Here's how the part is built. I have some questions about the finished solid (model axes, mm). A direction names the side the tool comes from. Coordinates: 2 decimals unless noted, no trailing zeros. Loops run counter-clockwise (first coordinate to the right, second up) from the corner with the lowest first, then second, coordinate; pieces in that order, holes last. Notation, with made-up numbers: (-23, -18) -> (-18, -18) arc R26 cw to (-18, 15) -> close; hole circle Ø7 at (21, -11.75). An arc over 180 degrees is marked (long way). Answer as a JSON object with one key per item and string values. Group by question number.
Q1. I want a section at A-A on z = 5. Count the separate pieces of the cut face and the enclosed holes in it, then the cut area to 3 significant figures.
Q2. I need wall thicknesses on line 1 (Z direction, x = -20.55, y = 65); line 2 (Y direction, x = -17.75, z = 3.5); line 3 (X direction, y = 22, z = 3.75). Which ranges of each line are inside material? Lowest first, please.
Q3. Thinking about a two-plate mould opening in Z: for faces 4 (the flat face through (-14, 39, 10)), 5 (the cylindrical face through (-19.96, 71.9, 5.09)), 6 (the flat face through (-17, 67, 3)), which applies, released by +Z, released by -Z, zero draft, split by the parting line, or undercut?
Q4. I'm going to push flat-ended pins straight in: pin 1 (3 mm diameter, centred on y = 40, z = 5.5, fed in from -X); pin 2 (3.5 mm diameter, centred on y = 65, z = 5, fed in from +X); pin 3 (6 mm diameter, centred on y = 21.5, z = 6, fed in from -X). Where does each tip first touch, or does it pass through?
Q5. On a 3-axis mill with a long thin cutter (end or side, diameter ignored), from which of +Z, -Z, +X, -X, +Y, -Y can I reach the whole of each face in a straight line? I mean faces 1 (the flat face through (-15, 20, 5)), 2 (the flat face through (-9.789, 2.098, 4.93)), 3 (the cylindrical face through (-22.4, 79.43, 5.07)). Say none if no direction works.
Q6. I want a section at C-C on x = -17.75. Write out the boundary of the cut face in (y, z).
Q7. I want a section at B-B on y = 66. Write out the boundary of the cut face in (x, z).
```python
from build123d import *

# Parameters (mm, degrees)
EXTRUDE_1_DEPTH     = 10
SKETCH_2_R          = 2.1
CUT_EXTRUDE_1_DEPTH = 82.018516402
SKETCH_3_R          = 0.8
CUT_EXTRUDE_2_DEPTH = 84.839131675
FILLET_1_R          = 0.5
FILLET_2_R          = 2


with BuildPart() as part:
    # 草图1 → 凸台-拉伸1 (new body)
    with BuildSketch(Plane.XY):
        Polygon((-9, 3.464101615), (-11, 0), (-9, -3.464101615), (-15, -3.464101615), (-15, 41.143593539), (-23, 55), (-23, 80), (-17, 80), (-17, 54.607695155), (-9, 40.751288694), align=None)
    extrude(amount=EXTRUDE_1_DEPTH)

    # 草图2 → 切除-拉伸1 (cut, through all)
    with BuildSketch(Plane(origin=(-17, 0, 0), x_dir=(0, 0, -1), z_dir=(1, 0, 0))):
        with Locations(Location((-5, 65, 0), (0, 0, 90))):
            Circle(SKETCH_2_R)
        with Locations(Location((-5, 74, 0), (0, 0, 90))):
            Circle(SKETCH_2_R)
    extrude(amount=-CUT_EXTRUDE_1_DEPTH, mode=Mode.SUBTRACT)

    # 草图3 → 切除-拉伸2 (cut, through all)
    with BuildSketch(Plane.XY.offset(10)):
        with Locations((-10.2, 0)):
            Circle(SKETCH_3_R)
        Polygon((-15, -1.07179677), (-13.618802154, -3.464101615), (-15, -3.464101615), align=None)
    extrude(amount=-CUT_EXTRUDE_2_DEPTH, mode=Mode.SUBTRACT)

    # 圆角1
    fillet_1_edges = [part.edges().sort_by_distance(p)[0] for p in [
        (-9, -3.464101615, 5),
        (-15, -1.07179677, 5),
        (-13.618802154, -3.464101615, 5),
    ]]
    fillet(fillet_1_edges, radius=FILLET_1_R)

    # 圆角2
    fillet_2_edges = [part.edges().sort_by_distance(p)[0] for p in [
        (-15, 41.143593539, 5),
        (-23, 55, 5),
        (-23, 80, 5),
        (-17, 80, 5),
        (-17, 54.607695155, 5),
        (-9, 40.751288694, 5),
    ]]
    fillet(fillet_2_edges, radius=FILLET_2_R)


solid = part.part
```
Result set:
{
 "1": {"separate pieces": "3", "enclosed holes": "0", "area": "437 mm²"},
 "2": {"line 1": "z = 0 to 2.9, 7.1 to 10", "line 2": "y = 45.91 to 63.53, 66.47 to 72.53, 75.47 to 79.56", "line 3": "x = -15 to -9"},
 "3": {"face 4": "released by +Z", "face 5": "undercut", "face 6": "zero draft"},
 "4": {"pin 1": "stops at x = -15.21", "pin 2": "passes through", "pin 3": "stops at x = -15"},
 "5": {"face 1": "+Z, -Z, -X, -Y", "face 2": "+Z, -Z, +X", "face 3": "+Z, -Z, -X, +Y"},
 "6": {"outline": "(45.91, 0) -> (79.56, 0) -> (79.56, 10) -> (45.91, 10) -> close; hole circle Ø4.2 at (65, 5); hole circle Ø4.2 at (74, 5)"},
 "7": {"outline": "(-23, 0) -> (-17, 0) -> (-17, 3.15) -> (-23, 3.15) -> close; (-23, 6.85) -> (-17, 6.85) -> (-17, 10) -> (-23, 10) -> close"}
}
